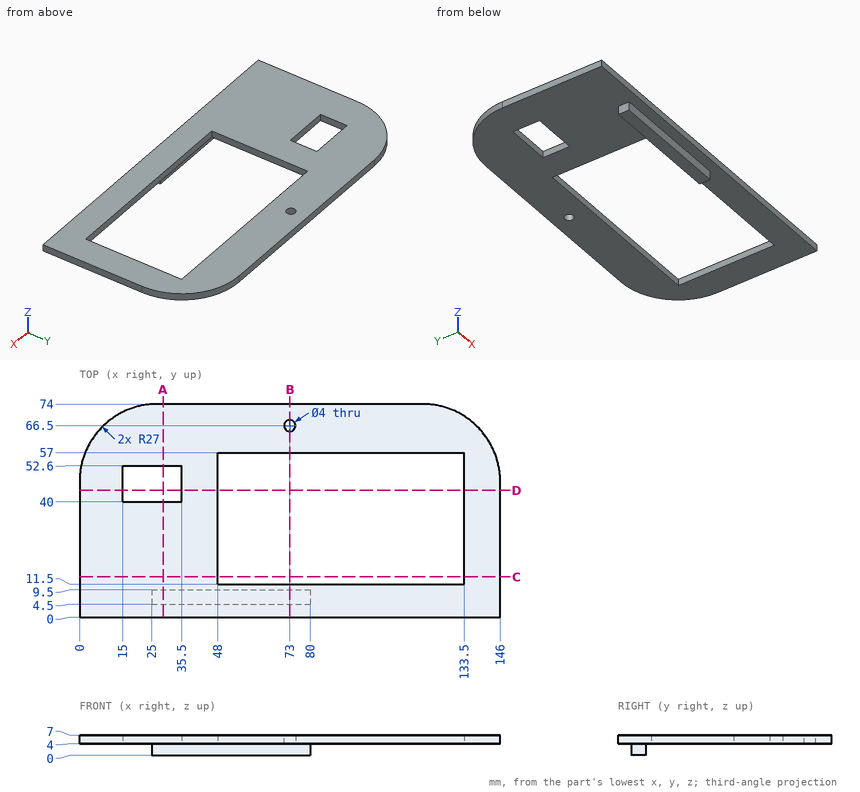
Job drawing, mm, ordinate dimensions from the low corner. One solid piece. Round coordinates to 2 decimals unless told otherwise and drop trailing zeros. Write each loop counter-clockwise with the first axis right and the second up, starting at its lowest first coordinate (ties: lowest second). Pieces come first, ordered by that corner, then holes. Notation, with made-up numbers: (28, -23) -> (55, -23) arc R7 ccw to (55, -16) -> close; hole circle Ø3 at (51.25, 33). An arc over 180 degrees is marked (long way). Answer as a JSON object with one key per item and string values.
(1) Band-saw the part on C-C, the plane y = 14. List the corners of the cut face in (x, z).
Reported:
{"outline": "(0, 4) -> (48, 4) -> (48, 7) -> (0, 7) -> close; (133.5, 4) -> (146, 4) -> (146, 7) -> (133.5, 7) -> close"}
(2) Pin check, flat tips, straight feed: P1, Ø1.5, axis at y = 48, z = 6, coming from the +X side; P2, Ø2, axis at y = 7.5, z = 2.5, coming from the +X side; P3, Ø1.2, axis at y = 8, z = 1, coming from the -X side. Stop position of each tip, or through.
Reported:
{"P1": "stops at x = 146", "P2": "stops at x = 80", "P3": "stops at x = 25"}
(3) Probe probe 1 along Y at (x, z) = (73, 4.8); probe 2 along X at (y, z) = (46, 4.75); probe 3 along Y at (x, z) = (52, 5.5). List the from-to ranges inside material, lowest first. Write a range as [from, to].
Reported:
{"probe 1": "y = [0, 11.5], [57, 64.5], [68.5, 74]", "probe 2": "x = [0, 15], [35.5, 48], [133.5, 146]", "probe 3": "y = [0, 11.5], [57, 74]"}
(4) Band-saw the part on D-D, the plane y = 44. List the corners of the cut face in (x, z), then the cut area to 3 significant figures.
Reported:
{"outline": "(0, 4) -> (15, 4) -> (15, 7) -> (0, 7) -> close; (35.5, 4) -> (48, 4) -> (48, 7) -> (35.5, 7) -> close; (133.5, 4) -> (146, 4) -> (146, 7) -> (133.5, 7) -> close", "area": "120 mm^2"}
(5) Band-saw the part on A-A, the plane x = 29. List the corners of the cut face in (y, z), then the cut area to 3 significant figures.
Reported:
{"outline": "(0, 4) -> (4.5, 4) -> (4.5, 0) -> (9.5, 0) -> (9.5, 4) -> (40, 4) -> (40, 7) -> (0, 7) -> close; (52.6, 4) -> (74, 4) -> (74, 7) -> (52.6, 7) -> close", "area": "204 mm^2"}
(6) Band-saw the part on B-B, the plane x = 73. List the corners of the cut face in (y, z), then the cut area to 3 significant figures.
Reported:
{"outline": "(0, 4) -> (4.5, 4) -> (4.5, 0) -> (9.5, 0) -> (9.5, 4) -> (11.5, 4) -> (11.5, 7) -> (0, 7) -> close; (57, 4) -> (64.5, 4) -> (64.5, 7) -> (57, 7) -> close; (68.5, 4) -> (74, 4) -> (74, 7) -> (68.5, 7) -> close", "area": "93.5 mm^2"}
